The drawing under review shows one solid part. Ordinate dimensions are in mm from its lowest x, y, z. A direction names the side the tool comes from. Coordinates: 2 decimals unless noted, no trailing zeros. Write each loop counter-clockwise with the first axis right and the second up, starting at its lowest first coordinate (ties: lowest second). Pieces come first, ordered by that corner, then holes.
1) For the marked faces 1 and 2, list the 3-axis set-ups (+Z, -Z, +X, -X, +Y, -Y) from which the entire face can be reached by the end or side of a thin tool; tool diameter is ignored.
2) Insertion check: P1, Ø4.5, axis at x = 102, z = 15, coming from the -Y side; P2, Ø7, axis at x = 15, y = 7.5, coming from the +Z side; P3, Ø9.5, axis at x = 95, y = 7.5, coming from the -Z side; P4, Ø3, axis at x = 43.5, y = 12.5, coming from the +Z side. Each pin has a flat end and moves straight along its axis. Give the tip position at first contact, or say it passes through.
3) We need section A-A on z = 16.5. Write out the cut boundary in (x, y), then the cut area to 3 significant figures.
4) We need section C-C on x = 66. Write out the cut boundary in (y, z), then the cut area to 3 significant figures.
5) We need section D-D on z = 5.5. Write out the cut boundary in (x, y).
6) We need section B-B on x = 95. Write out the cut boundary in (y, z), then the cut area to 3 significant figures.
7) To check wall thickness, follow line 1 along X through (y, z) = (15.6, 15); line 2 along Z through (x, y) = (26, 9); line 3 along Y through (x, z) = (78, 9.5). State the ranges of each line that lie inside material, in increasing order.
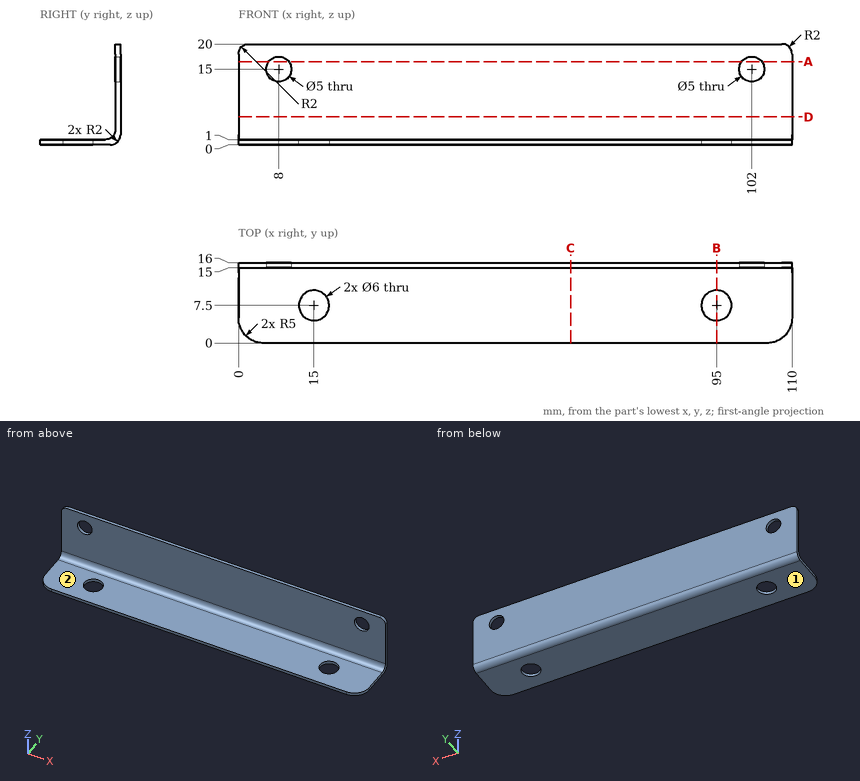
Result:
1. face 1: -Z, +X, -X, +Y, -Y
1. face 2: +Z, +X, -X, -Y
2. P1: passes through
2. P2: stops at z = 1
2. P3: stops at z = 0
2. P4: stops at z = 1.27
3. outline: (0, 15) - (6, 15) - (6, 16) - (0, 16) - close; (10, 15) - (100, 15) - (100, 16) - (10, 16) - close; (104, 15) - (110, 15) - (110, 16) - (104, 16) - close
3. area: 102 mm2
4. outline: (0, 0) - (14, 0) arc R2 ccw to (16, 2) - (16, 20) - (15, 20) - (15, 3) arc R2 cw to (13, 1) - (0, 1) - close
4. area: 35.0 mm2
5. outline: (0, 15) - (110, 15) - (110, 16) - (0, 16) - close
6. outline: (0, 0) - (4.5, 0) - (4.5, 1) - (0, 1) - close; (10.5, 0) - (14, 0) arc R2 ccw to (16, 2) - (16, 20) - (15, 20) - (15, 3) arc R2 cw to (13, 1) - (10.5, 1) - close
6. area: 29.0 mm2
7. line 1: x = 0 to 5.5, 10.5 to 99.5, 104.5 to 110
7. line 2: z = 0 to 1
7. line 3: y = 15 to 16
